Check sheet for the modelled part. Datum: model origin and axes. Units: mm. Face numbers are marked on the shaded views. A direction names the side the tool comes from. Give positions to 0.01 mm unless a question says otherwise; leave off trailing zeros. Order: outer loops, then holes, each group sorted by start corner. A loop starts at its lowest first (then second) coordinate and runs counter-clockwise, first axis right, second up. Notation, with made-up numbers: (7, 27.25) - (66, 27.25) arc R18 cw to (66, 44.25) - close; hole circle Ø8 at (-26.75, -37). An arc over 180 degrees is marked (long way). Answer in a Markdown table with one row per item.
Autodesk Inventor part; units mm, degrees
ref_plane "Work Plane1" through (0, 0, -15.0622) normal (0, 0, -1) x (-1, 0, 0)
ref_plane "Work Plane2" through (0, 0, -12.3) normal (0, 0, -1) x (-1, 0, 0)
ref_plane "YZ Plane" through (0, 0, 0) normal (1, 0, 0) x (0, 1, 0)
sketch "Sketch1" plane through (0, 0, 0) normal (0, 0, 1) x (1, 0, 0)
  circle A0 centre (0, 0) radius 1.5875
  dimension "d0" = 3.175
extrude "Extrusion1" add sketch "Sketch1" along normal mid plane 31.75
sketch "Sketch2" plane through (0, 0, 15.875) normal (0, 0, 1) x (1, 0, 0)
  circle A0 centre (0, 0) radius 1.4224
  dimension "d3" = 2.8448
extrude "Extrusion2" add sketch "Sketch2" along normal blind 5.715
ref_plane "Work Plane1" through (0, 0, -15.0622) normal (0, 0, -1) x (-1, 0, 0)
sketch "Sketch3" plane through (0, 0, -15.0622) normal (0, 0, -1) x (-1, 0, 0)
  circle A0 centre (0, 0) radius 1.4224
  circle A1 centre (0, 0) radius 1.5875
extrude "Extrusion3" cut sketch "Sketch3" against normal blind 0.381
ref_plane "Work Plane2" through (0, 0, -12.3) normal (0, 0, -1) x (-1, 0, 0)
sketch "Sketch4" plane through (0, 0, -12.3) normal (0, 0, -1) x (-1, 0, 0)
  circle A0 centre (0, 0) radius 1.4224
  circle A1 centre (0, 0) radius 1.5875
extrude "Extrusion4" cut sketch "Sketch4" against normal blind 0.381
chamfer "Chamfer1" distance 0.381 angle 45 2 edges at (-1.5875, 0, -15.875) (-1.4224, 0, 21.59)
thread "Thread1"
properties part number "Shock Shaft"
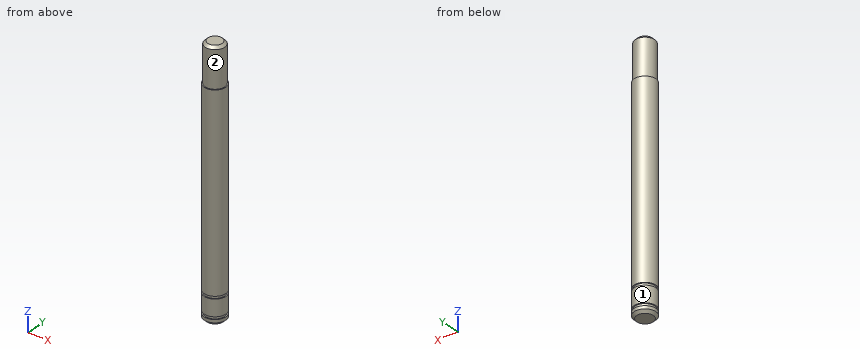
(1) Cross-section at C-C, the plane z = 2. Record the cut outline in (x, y) (1 decimal), then the cut area to 3 significant figures.
Geometry says:
| item | result |
|---|---|
| outline | circle Ø3.2 at (0, 0) |
| area | 7.92 mm² |
(2) Access from +Z, -Z, +X, -X, +Y, -Y to the whole of each face (thin tool, end or side, straight path). Record for the marked faces 1 and 2.
Geometry says:
| item | result |
|---|---|
| face 1 | +Z, -Z |
| face 2 | +Z |
(3) Gauge pin test, flat end, axial feed: P1, Ø1.5, axis at y = 1, z = -7, coming from the -X side. Record the tip position at first contact, or that the pin passes through.
Geometry says:
| item | result |
|---|---|
| P1 | x = -1.57 |
(4) Thickness scan on L1, parallel to Z at x = -1.3, y = -0.65 (3 decimals); L2, parallel to Y at x = 0.15, z = -7; L3, parallel to Y at x = 0.75, z = 16. Record the ranges inside material, lowest first.
Geometry says:
| item | result |
|---|---|
| L1 | -15.628 to -15.062, -14.681 to -12.3, -11.919 to 15.875 |
| L2 | -1.58 to 1.58 |
| L3 | -1.21 to 1.21 |
